```python
from build123d import *

# Parameters (mm, degrees)
F0_R     = 60
F1_DEPTH = 2.5
F2_R     = 1.4
F3_DEPTH = 12.5
F2_R_2   = 4
F4_DEPTH = 5.3
F6_DEPTH = 2.8
F7_R     = 2
F8_R     = 1


with BuildPart() as f1:
    # F0 (on Top) → F1 (new body)
    with BuildSketch(Plane.XY):
        Circle(F0_R)
    extrude(amount=F1_DEPTH)

    # F2 (on face) → F3 (cut, symmetric)
    with BuildSketch(Plane(origin=(0, 0, 0), x_dir=(1, 0, 0), z_dir=(0, 0, -1))):
        with Locations((0, -45)):
            Circle(F2_R)
        with Locations((-45, 0)):
            Circle(F2_R)
        with Locations((0, 45)):
            Circle(F2_R)
        with Locations((45, 0)):
            Circle(F2_R)
    extrude(amount=F3_DEPTH, both=True, mode=Mode.SUBTRACT)

    # F2 (on face) → F4 (join)
    with BuildSketch(Plane(origin=(0, 0, 0), x_dir=(1, 0, 0), z_dir=(0, 0, -1))):
        with Locations((-45, 0)):
            Circle(F2_R_2)
        with Locations((-45, 0)):
            Circle(F2_R, mode=Mode.SUBTRACT)
        with Locations((0, -45)):
            Circle(F2_R_2)
        with Locations((0, -45)):
            Circle(F2_R, mode=Mode.SUBTRACT)
        with Locations((45, 0)):
            Circle(F2_R_2)
        with Locations((45, 0)):
            Circle(F2_R, mode=Mode.SUBTRACT)
        with Locations((0, 45)):
            Circle(F2_R_2)
        with Locations((0, 45)):
            Circle(F2_R, mode=Mode.SUBTRACT)
    extrude(amount=-F4_DEPTH)

    # F5 (on face) → F6 (join)
    with BuildSketch(Plane.XY.offset(2.5)):
        with BuildLine():
            ThreePointArc((2.0400320513, 15.25), (2.4361318862, 15.8801411608), (2.8481367178, 16.5))
            Line((2.8481367178, 16.5), (-13, 16.5))
            Line((-13, 16.5), (-13, -16.5))
            Line((-13, -16.5), (2.8481367178, -16.5))
            ThreePointArc((2.8481367178, -16.5), (2.4361318862, -15.8801411608), (2.0400320513, -15.25))
            Line((2.0400320513, -15.25), (-11.75, -15.25))
            Line((-11.75, -15.25), (-11.75, 15.25))
            Line((-11.75, 15.25), (2.0400320513, 15.25))
        make_face()
        with BuildLine():
            ThreePointArc((3.5172935972, 15.25), (3.939229747, 15.8808335844), (4.3781079483, 16.5))
            Line((4.3781079483, 16.5), (2.8481367178, 16.5))
            ThreePointArc((2.8481367178, 16.5), (2.4361318862, 15.8801411608), (2.0400320513, 15.25))
            Line((2.0400320513, 15.25), (3.5172935972, 15.25))
        make_face()
        with BuildLine():
            Line((2.8481367178, -16.5), (4.3781079483, -16.5))
            ThreePointArc((4.3781079483, -16.5), (3.939229747, -15.8808335844), (3.5172935972, -15.25))
            Line((3.5172935972, -15.25), (2.0400320513, -15.25))
            ThreePointArc((2.0400320513, -15.25), (2.4361318862, -15.8801411608), (2.8481367178, -16.5))
        make_face()
        with BuildLine():
            ThreePointArc((3.5172935972, -15.25), (-1, 0), (3.5172935972, 15.25))
            Line((3.5172935972, 15.25), (2.0400320513, 15.25))
            ThreePointArc((2.0400320513, 15.25), (-2.25, 0), (2.0400320513, -15.25))
            Line((2.0400320513, -15.25), (3.5172935972, -15.25))
        make_face()
    extrude(amount=F6_DEPTH)

    # F7
    f7_edges = [f1.edges().sort_by_distance(p)[0] for p in [
        (4.378108, 16.5, 3.9),
        (4.378108, -16.5, 3.9),
    ]]
    fillet(f7_edges, radius=F7_R)

    # F8
    f8_edges = [f1.edges().sort_by_distance(p)[0] for p in [
        (2.040032, -15.25, 3.9),
        (2.040032, 15.25, 3.9),
        (-13, -16.5, 3.9),
        (-13, 16.5, 3.9),
    ]]
    fillet(f8_edges, radius=F8_R)


solid = f1.part
```
For this review, take the finished solid that the model builds, in its own axes (mm). A direction names the side the tool comes from. Round coordinates to 2 decimals unless told otherwise and drop trailing zeros. Write each loop counter-clockwise with the first axis right and the second up, starting at its lowest first coordinate (ties: lowest second). Pieces come first, ordered by that corner, then holes. Notation, with made-up numbers: (14.25, 51) - (72.25, 51) arc R12 ccw to (72.25, 69) - close; hole circle Ø2 at (-2, 62). An arc over 180 degrees is marked (long way). Answer as CSV lines item,"result". Start each with the question number.
(1) For line 1 (Y direction, x = 0, z = 1.9); line 2 (Y direction, x = -45, z = 4.1); line 3 (Z direction, x = 13.5, y = -43), list the stretches that pass through material, from the lowest coordinate up.
(2) Mouldability with a two-part tool opening along X and no side actions: class faces 1 (the cylindrical face through (-43.665, -0.421, 2.613)), 2 (the flat face through (-6, 16.5, 4)) as +X half, -X half, draft (parallel to the pull), parting line (faces both ways), or undercut.
(3) Add section A-A, the plane y = 0. State the section outline as (x, z) points.
(4) Add section C-C, the plane x = -45. State the section outline as (y, z) points, plus the area to 3 significant figures.
(5) For pin 1 (3 mm diameter, centred on x = 45, z = 2, fed in from +Y); pin 2 (2 mm diameter, centred on x = -4, z = 4.5, fed in from -Y); pin 3 (0.8 mm diameter, centred on y = -1.5, z = 3.5, fed in from -X); pin 4 (1.7 mm diameter, centred on x = 45, y = 0, fed in from -Z), all flat-tipped, find the tip position at first contact; note any pin that passes through.
(6) Add section D-D, the plane x = -8.5. State the section outline as (y, z) points.
(7) Machinability: for faces 3 (the flat face through (-6, -16.5, 4)), 4 (the flat face through (-13, 0, 4)), 5 (the flat face through (-6, -15.25, 4)), which of the approach directions +Z, -Z, +X, -X, +Y, -Y give a long, thin tool a straight path to every point of the face, cutting with its end or side? Answer none if there is none.
(8) Add section B-B, the plane z = 0.95. State the section outline as (x, y) points, plus the area to 3 significant figures.
From the geometry:
1,line 1,"y = -60 to -46.4, -43.6 to 43.6, 46.4 to 60"
1,line 2,"y = -4 to -1.4, 1.4 to 4"
1,line 3,"z = 0 to 2.5"
2,face 1,"undercut"
2,face 2,"draft"
3,outline,"(-60, 0) - (-46.4, 0) - (-46.4, 5.3) - (-49, 5.3) - (-49, 2.5) - (-60, 2.5) - close; (-43.6, 0) - (43.6, 0) - (43.6, 5.3) - (41, 5.3) - (41, 2.5) - (-1, 2.5) - (-1, 5.3) - (-2.25, 5.3) - (-2.25, 2.5) - (-11.75, 2.5) - (-11.75, 5.3) - (-13, 5.3) - (-13, 2.5) - (-41, 2.5) - (-41, 5.3) - (-43.6, 5.3) - close; (46.4, 0) - (60, 0) - (60, 2.5) - (49, 2.5) - (49, 5.3) - (46.4, 5.3) - close"
4,outline,"(-39.69, 0) - (-1.4, 0) - (-1.4, 5.3) - (-4, 5.3) - (-4, 2.5) - (-39.69, 2.5) - close; (1.4, 0) - (39.69, 0) - (39.69, 2.5) - (4, 2.5) - (4, 5.3) - (1.4, 5.3) - close"
4,area,"206 mm²"
5,pin 1,"stops at y = 41.32"
5,pin 2,"stops at y = -47.65"
5,pin 3,"stops at x = -48.85"
5,pin 4,"passes through"
6,outline,"(-59.39, 0) - (59.39, 0) - (59.39, 2.5) - (16.5, 2.5) - (16.5, 5.3) - (15.25, 5.3) - (15.25, 2.5) - (-15.25, 2.5) - (-15.25, 5.3) - (-16.5, 5.3) - (-16.5, 2.5) - (-59.39, 2.5) - close"
7,face 3,"+Z, +X, -X"
7,face 4,"+Z, +Y, -Y"
7,face 5,"+Z"
8,outline,"circle Ø120 at (0, 0); hole circle Ø2.8 at (-45, 0); hole circle Ø2.8 at (0, -45); hole circle Ø2.8 at (0, 45); hole circle Ø2.8 at (45, 0)"
8,area,"11,300 mm²"
